The listing builds one solid part. Answer for the finished solid, in the listing's coordinates (mm). A direction names the side the tool comes from. Coordinates: 2 decimals unless noted, no trailing zeros. Order: outer loops, then holes, each group sorted by start corner. A loop starts at its lowest first (then second) coordinate and runs counter-clockwise, first axis right, second up.
Autodesk Fusion 360 part; units mm, degrees
sketch "Skizze1" plane through (0, 0, 0) normal (0, 0, 1) x (1, 0, 0)
  line L0 (67.5, -18) -> (-67.5, -18)
  line L1 (-67.5, -18) -> (-67.5, 18)
  line L2 (-67.5, 18) -> (67.5, 18)
  line L3 (67.5, 18) -> (67.5, -18)
  line L4 (67.5, -18) -> (-67.5, 18) construction
  line L5 (-67.5, -18) -> (67.5, 18) construction
  line L6 (-73.8697, 0) -> (79.3057, 0) construction
  line L7 (-75.373, 13.97) -> (76.9673, 13.97) construction
  line L8 (-75.54, -13.97) -> (74.2946, -13.97) construction
  line L9 (-11, 24.3178) -> (-11, -28.2997) construction
  line L10 (-33, 24.986) -> (-33, -31.4735) construction
  line L11 (-55, 24.4848) -> (-55, -28.1327) construction
  line L12 (11, 24.8189) -> (11, -31.4735) construction
  line L13 (33, 24.6519) -> (33, -30) construction
  line L14 (55, 24.8189) -> (55, -30) construction
  circle A0 centre (-55, 0) radius 12.2
  circle A1 centre (-33, 0) radius 12.2
  circle A2 centre (-11, 0) radius 12.2
  circle A3 centre (11, 0) radius 12.2
  circle A4 centre (33, 0) radius 12.2
  circle A5 centre (55, 0) radius 12.2
  circle A6 centre (-55, 13.97) radius 4.2
  circle A7 centre (-33, 13.97) radius 4.2
  circle A8 centre (-11, 13.97) radius 4.2
  circle A9 centre (11, 13.97) radius 4.2
  circle A10 centre (33, 13.97) radius 4.2
  circle A11 centre (55, 13.97) radius 4.2
  circle A12 centre (-55, -13.97) radius 4.2
  circle A13 centre (-33, -13.97) radius 4.2
  circle A14 centre (-11, -13.97) radius 4.2
  circle A15 centre (11, -13.97) radius 4.2
  circle A16 centre (33, -13.97) radius 4.2
  circle A17 centre (55, -13.97) radius 4.2
  circle A18 centre (-55, 0) radius 9.25
  circle A19 centre (-33, 0) radius 9.25
  circle A20 centre (-11, 0) radius 9.25
  circle A21 centre (11, 0) radius 9.25
  circle A22 centre (33, 0) radius 9.25
  circle A23 centre (55, 0) radius 9.25
  line L15 (-51.75, -4.25) -> (-58.25, -4.25)
  line L16 (-58.25, -4.25) -> (-58.25, 4.25)
  line L17 (-58.25, 4.25) -> (-51.75, 4.25)
  line L18 (-51.75, 4.25) -> (-51.75, -4.25)
  line L19 (-51.75, -4.25) -> (-58.25, 4.25) construction
  line L20 (-58.25, -4.25) -> (-51.75, 4.25) construction
  line L21 (-29.75, -4.25) -> (-36.25, -4.25)
  line L22 (-36.25, -4.25) -> (-36.25, 4.25)
  line L23 (-36.25, 4.25) -> (-29.75, 4.25)
  line L24 (-29.75, 4.25) -> (-29.75, -4.25)
  line L25 (-29.75, -4.25) -> (-36.25, 4.25) construction
  line L26 (-36.25, -4.25) -> (-29.75, 4.25) construction
  line L27 (-7.75, -4.25) -> (-14.25, -4.25)
  line L28 (-14.25, -4.25) -> (-14.25, 4.25)
  line L29 (-14.25, 4.25) -> (-7.75, 4.25)
  line L30 (-7.75, 4.25) -> (-7.75, -4.25)
  line L31 (-7.75, -4.25) -> (-14.25, 4.25) construction
  line L32 (-14.25, -4.25) -> (-7.75, 4.25) construction
  line L33 (14.25, -4.25) -> (7.75, -4.25)
  line L34 (7.75, -4.25) -> (7.75, 4.25)
  line L35 (7.75, 4.25) -> (14.25, 4.25)
  line L36 (14.25, 4.25) -> (14.25, -4.25)
  line L37 (14.25, -4.25) -> (7.75, 4.25) construction
  line L38 (7.75, -4.25) -> (14.25, 4.25) construction
  line L39 (36.25, -4.25) -> (29.75, -4.25)
  line L40 (29.75, -4.25) -> (29.75, 4.25)
  line L41 (29.75, 4.25) -> (36.25, 4.25)
  line L42 (36.25, 4.25) -> (36.25, -4.25)
  line L43 (36.25, -4.25) -> (29.75, 4.25) construction
  line L44 (29.75, -4.25) -> (36.25, 4.25) construction
  line L45 (58.25, -4.25) -> (51.75, -4.25)
  line L46 (51.75, -4.25) -> (51.75, 4.25)
  line L47 (51.75, 4.25) -> (58.25, 4.25)
  line L48 (58.25, 4.25) -> (58.25, -4.25)
  line L49 (58.25, -4.25) -> (51.75, 4.25) construction
  line L50 (51.75, -4.25) -> (58.25, 4.25) construction
  line L51 (-60.5, 33.1976) -> (-60.5, -30) construction
  line L52 (-89, -7) -> (78, -7) construction
  line L53 (-60.5, -18) -> (-67.5, -7)
  line L54 (60.5, 21.7982) -> (60.5, -34.2962) construction
  line L55 (60.5, -18) -> (67.5, -7)
  point P0 (-55, 0)
  point P1 (-33, 0)
  point P2 (-11, 0)
  point P3 (11, 0)
  point P4 (33, 0)
  point P5 (55, 0)
  dimension "d1" = 135
  dimension "d2" = 36
  dimension "d3" = 13.97
  dimension "d4" = 13.97
  dimension "d5" = 11
  dimension "d6" = 11
  dimension "d7" = 22
  dimension "d8" = 22
  dimension "d9" = 22
  dimension "d10" = 22
  dimension "d11" = 24.4
  dimension "d12" = 24.4
  dimension "d13" = 24.4
  dimension "d14" = 24.4
  dimension "d15" = 24.4
  dimension "d16" = 24.4
  dimension "d17" = 8.4
  dimension "d18" = 8.4
  dimension "d19" = 8.4
  dimension "d20" = 8.4
  dimension "d21" = 8.4
  dimension "d22" = 8.4
  dimension "d23" = 8.4
  dimension "d24" = 8.4
  dimension "d25" = 8.4
  dimension "d26" = 8.4
  dimension "d27" = 8.4
  dimension "d28" = 8.4
  dimension "d29" = 18.5
  dimension "d30" = 18.5
  dimension "d31" = 18.5
  dimension "d32" = 18.5
  dimension "d33" = 18.5
  dimension "d34" = 18.5
  dimension "d35" = 6.5
  dimension "d36" = 6.5
  dimension "d37" = 6.5
  dimension "d38" = 6.5
  dimension "d39" = 6.5
  dimension "d40" = 6.5
  dimension "d41" = 8.5
  dimension "d42" = 8.5
  dimension "d43" = 8.5
  dimension "d44" = 8.5
  dimension "d45" = 8.5
  dimension "d46" = 8.5
  dimension "d59" = 7
  dimension "d60" = 25
  dimension "d61" = 7
  dimension "d62" = 12.5
  dimension "d63" = 18
extrude "Extrusion2" add sketch "Skizze1" along normal blind 8.3 contours L0 L2 L3 A5 A11 A17 L55 | L0 A5 A17 | L0 A4 A5 A16 A17 | L2 A5 A11 | L0 A4 A16 | A5 A17 | A4 A5 A11 A17 | L2 A4 A5 A10 A11 | L0 A3 A4 A15 A16 | A4 A5 | A3 A4 A5 A10 A16 | L2 A4 A10 | A5 A11 | L0 A3 A15 | A4 A16 | L2 A3 A4 A9 A10 | L0 A2 A3 A14 A15 | A3 A4 | A2 A3 A4 A9 A15 | A4 A10 | L2 A3 A9 | L0 A2 A14 | A3 A15 | L2 A2 A3 A8 A9 | L0 A1 A2 A13 A14 | A2 A3 | A1 A2 A3 A8 A14 | A3 A9 | L2 A2 A8 | L0 A1 A13 | A2 A14 | L2 A1 A2 A7 A8 | L0 A0 A1 A12 A13 | A1 A2 | A0 A1 A2 A7 A13 | A2 A8 | L2 A1 A7 | L0 A0 A12 | A1 A13 | L2 A0 A1 A6 A7 | L0 L1 L2 A0 A6 A12 L53 | A0 A1 | A0 A1 A6 A12 | A1 A7 | L2 A0 A6 | A0 A12 | A0 A6 | A18 | A19 | A20 | A21 | A22 | A23 | L15 L16 L17 L18 | L21 L22 L23 L24 | L27 L28 L29 L30 | L33 L34 L35 L36 | L39 L40 L41 L42 | L45 L46 L47 L48
extrude "Extrusion3" cut sketch "Skizze1" along normal blind 9 contours L0 A5 A17 | L2 A5 A11 | L0 A4 A16 | A5 A17 | L2 A4 A10 | A5 A11 | L0 A3 A15 | A4 A16 | A4 A10 | L2 A3 A9 | L0 A2 A14 | A3 A15 | A3 A9 | L2 A2 A8 | L0 A1 A13 | A2 A14 | A2 A8 | L2 A1 A7 | L0 A0 A12 | A1 A13 | A1 A7 | L2 A0 A6 | A0 A12 | A0 A6
extrude "Extrusion4" cut sketch "Skizze1" along normal blind 4 contours A4 A5 A11 A17 | A4 A5 | A3 A4 A5 A10 A16 | A3 A4 | A2 A3 A4 A9 A15 | A2 A3 | A1 A2 A3 A8 A14 | A1 A2 | A0 A1 A2 A7 A13 | A0 A1 | A0 A1 A6 A12
extrude "Extrusion5" cut sketch "Skizze1" along normal blind 6 contours A18 | A19 | A20 | A21 | A22 | A23
extrude "Extrusion6" cut sketch "Skizze1" along normal blind 9 contours L15 L16 L17 L18 | L21 L22 L23 L24 | L27 L28 L29 L30 | L33 L34 L35 L36 | L39 L40 L41 L42 | L45 L46 L47 L48
(1) Find section D-D (y = -13.97). Write down the section's boundary in (x, z), and give its area (3 significant figures).
(2) Find section A-A (y = 13.97). Write down the section's boundary in (x, z).
(3) Find section B-B (x = 11). Write down the section's boundary in (y, z), and give its area (3 significant figures).
(4) For faces 5 (the face through (44, 18, 4)), 6 (the face through (-25.119, 9.313, 1.972)), 7 (the face through (-11, -4.25, 7)), determine the directions among +Z, -Z, +X, -X, +Y, -Y from which every point of the face is accessible in a straight line to the end or side of a thin tool.
(5) Each of these flat-tipped pins is pushed along its axis until it touches: pin 1 Ø5 at (x, y) = (-11, -13.97) entering from +Z (3 decimals); pin 2 Ø1 at (x, z) = (11.5, 7) entering from -Y; pin 3 Ø1.2 at (x, z) = (33, 6.5) entering from +Y. Where does it stop, or does it pass through?
(6) Consider line 1 (Y direction, x = -32.5, z = 5.25); line 2 (Z direction, x = 54, y = 5.5); line 3 (Y direction, x = 33, z = 6.5). Determine where each line is inside the solid, lowest interval first.
(7) The mould has two halves that part along X. Classify faces 1 (the face through (-51, 0, 6)), 2 (the face through (-2.455, 3.543, 4.986)), 3 (the face through (-63.95, -12.58, 4.09)), 4 (the face through (-67, 4, 0)): released by +X, released by -X, zero draft, split by the parting line, or undercut.
(8) Find section C-C (x = -17). Write down the section's boundary in (y, z), and give its area (3 significant figures).
Findings below:
1. outline: (-63.06, 0) - (-59.2, 0) - (-59.2, 8.3) - (-63.06, 8.3) - close; (-50.8, 0) - (-37.2, 0) - (-37.2, 8.3) - (-50.8, 8.3) - close; (-28.8, 0) - (-15.2, 0) - (-15.2, 8.3) - (-28.8, 8.3) - close; (-6.8, 0) - (6.8, 0) - (6.8, 8.3) - (-6.8, 8.3) - close; (15.2, 0) - (28.8, 0) - (28.8, 8.3) - (15.2, 8.3) - close; (37.2, 0) - (50.8, 0) - (50.8, 8.3) - (37.2, 8.3) - close; (59.2, 0) - (63.06, 0) - (63.06, 8.3) - (59.2, 8.3) - close
1. area: 629 mm2
2. outline: (-67.5, 0) - (-59.2, 0) - (-59.2, 8.3) - (-67.5, 8.3) - close; (-50.8, 0) - (-37.2, 0) - (-37.2, 8.3) - (-50.8, 8.3) - close; (-28.8, 0) - (-15.2, 0) - (-15.2, 8.3) - (-28.8, 8.3) - close; (-6.8, 0) - (6.8, 0) - (6.8, 8.3) - (-6.8, 8.3) - close; (15.2, 0) - (28.8, 0) - (28.8, 8.3) - (15.2, 8.3) - close; (37.2, 0) - (50.8, 0) - (50.8, 8.3) - (37.2, 8.3) - close; (59.2, 0) - (67.5, 0) - (67.5, 8.3) - (59.2, 8.3) - close
3. outline: (-9.77, 4) - (-9.25, 4) - (-9.25, 6) - (-4.25, 6) - (-4.25, 8.3) - (-9.77, 8.3) - close; (4.25, 6) - (9.25, 6) - (9.25, 4) - (9.77, 4) - (9.77, 8.3) - (4.25, 8.3) - close
3. area: 27.5 mm2
4. face 5: +Z, -Z, +X, -X, +Y
4. face 6: -Z
4. face 7: +Z, -Z
5. pin 1: passes through
5. pin 2: stops at y = -9.89
5. pin 3: stops at y = 9.81
6. line 1: y = -9.8 to -9.24, 9.24 to 9.8
6. line 2: z = 6 to 8.3
6. line 3: y = -9.77 to -4.25, 4.25 to 9.77
7. face 1: undercut
7. face 2: undercut
7. face 3: released by -X
7. face 4: zero draft
8. outline: (-18, 0) - (-10.62, 0) - (-10.62, 4) - (-7.04, 4) - (-7.04, 6) - (7.04, 6) - (7.04, 4) - (10.62, 4) - (10.62, 0) - (18, 0) - (18, 8.3) - (-18, 8.3) - close
8. area: 186 mm2
